Can you work these out from the drawing? Everything is in mm from the part's minimum corner. A direction names the side the tool comes from. Round coordinates to 2 decimals unless told otherwise and drop trailing zeros. Order: outer loops, then holes, each group sorted by start corner. A loop starts at its lowest first (then second) coordinate and runs counter-clockwise, first axis right, second up. Notation, with made-up numbers: (36.25, 59.25) - (84.25, 59.25) arc R26 ccw to (84.25, 77.25) - close; hole circle Ø8 at (64, -7). An arc over 180 degrees is marked (long way). Answer as a JSON object with one key per item and string values.
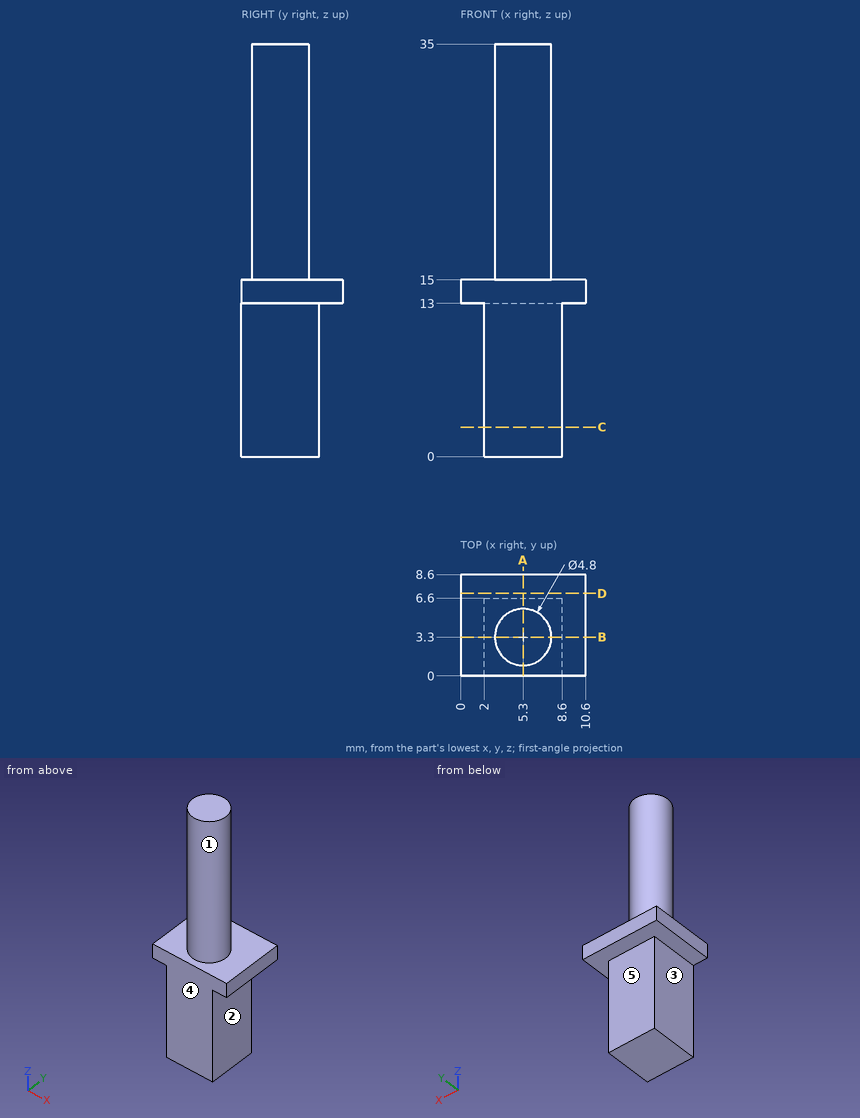
1. Imagine slicing it at D-D (y = 7). List the corners of the cut face in (x, z) for me, plus the area to 3 significant figures.
Responses:
{"outline": "(0, 13) - (10.6, 13) - (10.6, 15) - (0, 15) - close", "area": "21.2 mm2"}
2. Imagine slicing it at C-C (z = 2.5). List the corners of the cut face in (x, y) for me.
Responses:
{"outline": "(2, 0) - (8.6, 0) - (8.6, 6.6) - (2, 6.6) - close"}
3. For the marked faces 1, 2, 3, 4 and 5, which set-ups out of +Z, -Z, +X, -X, +Y, -Y let a thin tool reach every point of the face, with its end or its side?
Responses:
{"face 1": "+Z", "face 2": "-Z, +X, +Y, -Y", "face 3": "-Z, -X, +Y, -Y", "face 4": "+Z, -Z, +X, -X, -Y", "face 5": "-Z, +X, -X, +Y"}
4. If I drill on L1, parallel to Z at x = 10.25, y = 2.25; L2, parallel to Z at x = 7, y = 6.5; L3, parallel to Y at x = 8.25, z = 3, over which ranges is the centre line in solid material (lowest first)? Write a range as [from, to].
Responses:
{"L1": "[13, 15]", "L2": "[0, 15]", "L3": "[0, 6.6]"}
5. Imagine slicing it at A-A (x = 5.3). List the corners of the cut face in (y, z) for me, plus the area to 3 significant figures.
Responses:
{"outline": "(0, 0) - (6.6, 0) - (6.6, 13) - (8.6, 13) - (8.6, 15) - (5.7, 15) - (5.7, 35) - (0.9, 35) - (0.9, 15) - (0, 15) - close", "area": "199 mm2"}
6. Imagine slicing it at B-B (y = 3.3). List the corners of the cut face in (x, z) for me, plus the area to 3 significant figures.
Responses:
{"outline": "(0, 13) - (2, 13) - (2, 0) - (8.6, 0) - (8.6, 13) - (10.6, 13) - (10.6, 15) - (7.7, 15) - (7.7, 35) - (2.9, 35) - (2.9, 15) - (0, 15) - close", "area": "203 mm2"}
7. For P1, Ø3.5, axis at y = 5, z = 6, coming from the +X side; P2, Ø4, axis at y = 4.5, z = 26, coming from the +X side; P3, Ø1.5, axis at y = 1, z = 16, coming from the +X side, each with a flat end and sliding along its axis, tell me the tip position at first contact or that it passes through.
Responses:
{"P1": "x = 8.6", "P2": "x = 7.7", "P3": "x = 7.13"}
